Geometry check sheet. Reference: the model listing, model coordinates, mm. Round coordinates to 2 decimals unless told otherwise and drop trailing zeros. Loops run counter-clockwise (first coordinate to the right, second up) from the corner with the lowest first, then second, coordinate; pieces in that order, holes last. Notation, with made-up numbers: (32, 61) -> (70, 61) arc R5 ccw to (70, 68) -> close; hole circle Ø1 at (77.5, 64.25). An arc over 180 degrees is marked (long way). Use a Markdown table: item, result. Add a question column.
Q1. Sectioned sample at C-C, the plane x = 0. Enter the section's corners in (y, z).
Q2. Material ranges on L1, parallel to Y at x = 0, z = 1.8; L2, parallel to Y at x = -11, z = 2.8, recorded low to high.
Q3. Sectioned sample at B-B, the plane z = 0.95. Enter the section's corners in (x, y).
Q4. Release check for a two-part mould opening along Y. For faces 1 (the face through (-0.59, -41.74, 3.04)), 2 (the face through (-4.817, 210.285, 3.042)), 3 (the face through (-2, 3, 0)) record: released by +Y, released by -Y, zero draft, split by the parting line, or undercut.
Q5. Sectioned sample at A-A, the plane y = 173.6. Enter the section's corners in (x, z), then the cut area to 3 significant figures.
Q6. Sectioned sample at D-D, the plane y = -46.2. Enter the section's corners in (x, z).
Q7. Gauge pin test, flat end, axial feed: P1, Ø7, axis at x = 0, y = -46.2, coming from the -Z side. Record the tip position at first contact, or that the pin passes through.
```python
from build123d import *

# Parameters (mm, degrees)
SKETCH1_W           = 304.8
SKETCH1_H           = 457.2
BOSS_EXTRUDE1_DEPTH = 6
SKETCH2_R           = 37
CUT_EXTRUDE1_DEPTH  = 275.808515152
SKETCH3_R           = 4.5
CUT_EXTRUDE2_DEPTH  = 275.808515152


with BuildPart() as part:
    # Sketch1 → Boss-Extrude1 (new body)
    with BuildSketch(Plane.XY):
        Rectangle(SKETCH1_W, SKETCH1_H)
    extrude(amount=BOSS_EXTRUDE1_DEPTH)

    # Sketch2 → Cut-Extrude1 (cut, through all)
    with BuildSketch(Plane.XY.offset(6)):
        with Locations((0, 173.6)):
            Circle(SKETCH2_R)
    extrude(amount=-CUT_EXTRUDE1_DEPTH, mode=Mode.SUBTRACT)

    # Sketch3 → Cut-Extrude2 (cut, through all)
    with BuildSketch(Plane.XY.offset(6)):
        with Locations((0, -46.2)):
            Circle(SKETCH3_R)
    extrude(amount=-CUT_EXTRUDE2_DEPTH, mode=Mode.SUBTRACT)


solid = part.part
```
Values:
| question | item | result |
|---|---|---|
| 1 | outline | (-228.6, 0) -> (-50.7, 0) -> (-50.7, 6) -> (-228.6, 6) -> close; (-41.7, 0) -> (136.6, 0) -> (136.6, 6) -> (-41.7, 6) -> close; (210.6, 0) -> (228.6, 0) -> (228.6, 6) -> (210.6, 6) -> close |
| 2 | L1 | -228.6 to -50.7, -41.7 to 136.6, 210.6 to 228.6 |
| 2 | L2 | -228.6 to 138.27, 208.93 to 228.6 |
| 3 | outline | (-152.4, -228.6) -> (152.4, -228.6) -> (152.4, 228.6) -> (-152.4, 228.6) -> close; hole circle Ø74 at (0, 173.6); hole circle Ø9 at (0, -46.2) |
| 4 | face 1 | undercut |
| 4 | face 2 | undercut |
| 4 | face 3 | zero draft |
| 5 | outline | (-152.4, 0) -> (-37, 0) -> (-37, 6) -> (-152.4, 6) -> close; (37, 0) -> (152.4, 0) -> (152.4, 6) -> (37, 6) -> close |
| 5 | area | 1,380 mm^2 |
| 6 | outline | (-152.4, 0) -> (-4.5, 0) -> (-4.5, 6) -> (-152.4, 6) -> close; (4.5, 0) -> (152.4, 0) -> (152.4, 6) -> (4.5, 6) -> close |
| 7 | P1 | through |
